from build123d import *

# Parameters (mm, degrees)
SKETCH1_R           = 100
SKETCH1_R_2         = 79.286499618
SKETCH1_R_3         = 15
SKETCH1_R_4         = 10
BOSS_EXTRUDE1_DEPTH = 10


with BuildPart() as part:
    # Sketch1 → Boss-Extrude1 (new body)
    with BuildSketch(Plane(origin=(0, 0, 0), x_dir=(0, 0, -1), z_dir=(1, 0, 0))):
        Circle(SKETCH1_R)
        Circle(SKETCH1_R_2, mode=Mode.SUBTRACT)
        with BuildLine():
            Line((-5, -14.142135624), (-5, -79.128686465))
            ThreePointArc((-5, -79.128686465), (0, -79.286499618), (5, -79.128686465))
            Line((5, -79.128686465), (5, -14.142135624))
            ThreePointArc((5, -14.142135624), (0, -15), (-5, -14.142135624))
        make_face()
        with BuildLine():
            Line((-14.142135624, 5), (-79.128686465, 5))
            ThreePointArc((-79.128686465, 5), (-79.286499618, 0), (-79.128686465, -5))
            Line((-79.128686465, -5), (-14.142135624, -5))
            ThreePointArc((-14.142135624, -5), (-15, 0), (-14.142135624, 5))
        make_face()
        with BuildLine():
            ThreePointArc((5, 79.128686465), (0, 79.286499618), (-5, 79.128686465))
            Line((-5, 79.128686465), (-5, 14.142135624))
            ThreePointArc((-5, 14.142135624), (0, 15), (5, 14.142135624))
            Line((5, 14.142135624), (5, 79.128686465))
        make_face()
        with BuildLine():
            ThreePointArc((79.286499618, 0), (79.247036509, 2.50124494), (79.128686465, 5))
            Line((79.128686465, 5), (14.142135624, 5))
            ThreePointArc((14.142135624, 5), (14.783978395, 2.536529681), (15, 0))
            ThreePointArc((15, 0), (14.783978395, -2.536529681), (14.142135624, -5))
            Line((14.142135624, -5), (79.128686465, -5))
            ThreePointArc((79.128686465, -5), (79.247036509, -2.50124494), (79.286499618, 0))
        make_face()
        Circle(SKETCH1_R_3)
        Circle(SKETCH1_R_4, mode=Mode.SUBTRACT)
    extrude(amount=BOSS_EXTRUDE1_DEPTH)


solid = part.part
The model under review builds one solid part; all positions refer to its coordinate system, in mm. A direction names the side the tool comes from. Coordinates: 2 decimals unless noted, no trailing zeros. Loops run counter-clockwise (first coordinate to the right, second up) from the corner with the lowest first, then second, coordinate; pieces in that order, holes last.
(1) Insertion check: P1, Ø3, axis at x = 4.5, y = -33.5, coming from the -Z side; P2, Ø3, axis at x = 7, y = 32.5, coming from the +Z side; P3, Ø5, axis at x = 2.5, y = 43, coming from the -Z side. Each pin has a flat end and moves straight along its axis. Give the tip position at first contact, or say it passes through.
Determined:
P1: stops at z = -94.74
P2: stops at z = 95.07
P3: stops at z = -91.43
(2) Wall thickness on L1, parallel to Y at x = 7.5, z = -41; L2, parallel to Y at x = 3.75, z = 15.5; L3, parallel to Y at x = 7.5, z = 0: over which ranges is each line inside the solid? List them lowest first.
Determined:
L1: y = -91.21 to -67.86, -5 to 5, 67.86 to 91.21
L2: y = -98.79 to -77.76, -5 to 5, 77.76 to 98.79
L3: y = -100 to -10, 10 to 100
(3) Consider section A-A, the plane y = 0. Give the boundary of the cut face in (x, z).
Determined:
outline: (0, -100) - (10, -100) - (10, -10) - (0, -10) - close; (0, 10) - (10, 10) - (10, 100) - (0, 100) - close
(4) Consider section D-D, the plane y = 21.5. Give the boundary of the cut face in (x, z).
Determined:
outline: (0, -97.66) - (10, -97.66) - (10, -76.32) - (0, -76.32) - close; (0, -5) - (10, -5) - (10, 5) - (0, 5) - close; (0, 76.32) - (10, 76.32) - (10, 97.66) - (0, 97.66) - close
(5) Tool access review of faces 4 (the flat face through (5, 5, 46)), 5 (the flat face through (0, -21, 1)): name each direction out of +Z, -Z, +X, -X, +Y, -Y from which nothing blocks a thin tool from reaching the whole face with its end or side.
Determined:
face 4: +X, -X
face 5: +Z, -Z, -X, +Y, -Y
(6) Draft analysis for pull direction Y (two halves, no side actions). For faces 1 (the flat face through (10, -21, 1)), 2 (the cylindrical face through (4.93, 30.04, -95.38)), 3 (the cylindrical face through (4.93, 55.49, 56.63)), state which applies: +Y half, -Y half, draft (parallel to the pull), parting line (faces both ways), or undercut.
Determined:
face 1: draft
face 2: parting line
face 3: undercut
(7) Consider section C-C, the plane x = 6.5. Give the boundary of the cut face in (y, z).
Determined:
outline: circle Ø200 at (0, 0); hole (-79.13, -5) arc R79.29 ccw to (-5, -79.13) - (-5, -14.14) arc R15 cw to (-14.14, -5) - close; hole (-79.13, 5) - (-14.14, 5) arc R15 cw to (-5, 14.14) - (-5, 79.13) arc R79.29 ccw to start; hole circle Ø20 at (0, 0); hole (5, -79.13) arc R79.29 ccw to (79.13, -5) - (14.14, -5) arc R15 cw to (5, -14.14) - close; hole (5, 14.14) arc R15 cw to (14.14, 5) - (79.13, 5) arc R79.29 ccw to (5, 79.13) - close
